Design review of the part built by this model. Coordinates are the model's own, in mm. Give positions to 0.01 mm unless a question says otherwise; leave off trailing zeros. Write each loop counter-clockwise with the first axis right and the second up, starting at its lowest first coordinate (ties: lowest second). Pieces come first, ordered by that corner, then holes. Notation, with made-up numbers: (55, 18.5) -> (95, 18.5) arc R24 cw to (95, 41.5) -> close; hole circle Ø4 at (43.25, 63.25). An arc over 180 degrees is marked (long way). Write each question's results on one line, items separated by ' | '. Start each with the question number.
(1) Take a section at A-A (x = 0). State the section outline as (y, z) points (3 decimals), plus the area to 3 significant figures.
(2) Take a section at C-C (z = 0). State the section outline as (x, y) points (3 decimals), plus the area to 3 significant figures.
(3) To check wall thickness, follow probe 1 along Y at (x, z) = (0, 0) (3 decimals); probe 2 along X at (y, z) = (-2, 0.05); probe 3 along Y at (x, z) = (1.25, -0.3). State the ranges of each line that lie inside material, in increasing order.
Autodesk Inventor part; units mm, degrees
ref_plane "YZ Plane" through (0, 0, 0) normal (1, 0, 0) x (0, 1, 0)
ref_plane "XZ Plane" through (0, 0, 0) normal (0, 1, 0) x (-1, 0, 0)
ref_plane "XY Plane" through (0, 0, 0) normal (0, 0, 1) x (1, 0, 0)
sketch "Skizze1" plane through (0, 0, 0) normal (0, 0, 1) x (1, 0, 0)
  circle A0 centre (0, 0) radius 2.7
  circle A1 centre (0, 0) radius 3.325
  dimension "d0" = 5.4
  dimension "d1" = 6.65
extrude "Extrusion1" add sketch "Skizze1" along normal mid plane 1
fillet "Rundung1" radius 0.2 4 edges at (-3.325, 0, 0.5) (-3.325, 0, -0.5) (-2.7, 0, 0.5) (-2.7, 0, -0.5)
properties part number "YTP-AP-E20-R1.0" material "Gummi, Silikon"
Report:
1) outline: (-3.325, -0.3) arc R0.2 ccw to (-3.125, -0.5) -> (-2.9, -0.5) arc R0.2 ccw to (-2.7, -0.3) -> (-2.7, 0.3) arc R0.2 ccw to (-2.9, 0.5) -> (-3.125, 0.5) arc R0.2 ccw to (-3.325, 0.3) -> close; (2.7, -0.3) arc R0.2 ccw to (2.9, -0.5) -> (3.125, -0.5) arc R0.2 ccw to (3.325, -0.3) -> (3.325, 0.3) arc R0.2 ccw to (3.125, 0.5) -> (2.9, 0.5) arc R0.2 ccw to (2.7, 0.3) -> close | area: 1.18 mm2
2) outline: circle Ø6.65 at (0, 0); hole circle Ø5.4 at (0, 0) | area: 11.8 mm2
3) probe 1: -3.325 to -2.7, 2.7 to 3.325 | probe 2: -2.66 to -1.81, 1.81 to 2.66 | probe 3: -3.08 to -2.39, 2.39 to 3.08
